Design review of the part built by this model. Coordinates are the model's own, in mm. Coordinates: 2 decimals unless noted, no trailing zeros. Loops run counter-clockwise (first coordinate to the right, second up) from the corner with the lowest first, then second, coordinate; pieces in that order, holes last. Notation, with made-up numbers: (9, 31) - (29, 31) arc R31 ccw to (29, 68) - close; hole circle Ø9 at (89, -39). An arc over 180 degrees is marked (long way). Answer in a Markdown table with one row per item. Add a question column.
(1) We need section A-A, the plane z = 2.5. Give the number of separate pieces and of enclosed holes in the cut face, plus the area to 3 significant figures.
(2) The part is to be moulded in two halves that separate along Y. For faces 1 (the face through (48, -48, 10)), 2 (the face through (50, 39.979, 5)), 3 (the face through (106.06, 9.77, 4.93)), say which applies: released by +Y, released by -Y, zero draft, split by the parting line, or undercut.
(3) To check wall thickness, follow L1, parallel to X at y = -23, z = 9.25; L2, parallel to X at y = -48.5, z = 7.25; L3, parallel to Y at x = -9, z = 0.75. State the ranges of each line that lie inside material, in increasing order. Write a range as [from, to].
(4) Clearance check with flat-ended pins moving along their axes: pin 1 (5 mm diameter, centred on x = -10, y = -6.5, fed in from -Z); pin 2 (5 mm diameter, centred on x = 109.23, y = -109.52, fed in from -Z); pin 3 (11 mm diameter, centred on x = 49.23, y = -69.52, fed in from +Z); pin 4 (10 mm diameter, centred on x = 49.23, y = -29.52, fed in from +Z). State where each tip first meets the part, or that it passes through.
(5) We need section B-B, the plane y = -52.5. Write out the cut boundary in (x, z), plus the area to 3 significant figures.
Solid Edge part; units mm, degrees
sketch "Sketch1" plane through (0, 0, 0) normal (0, 0, 1) x (1, 0, 0)
  line L0 (-25.7684, -139.0211) -> (124.2316, -139.0211)
  line L1 (124.2316, -139.0211) -> (124.2316, 39.9789)
  line L2 (124.2316, 39.9789) -> (-25.7684, 39.9789)
  line L3 (-25.7684, 39.9789) -> (-25.7684, -139.0211)
extrude "Protrusion1" add sketch "Sketch1" along normal blind 10
sketch "Sketch2" plane through (49.2316, -49.5211, 10) normal (0, 0, 1) x (0, -1, 0)
  circle A0 centre (0, 45) radius 15
extrude "Cutout1" cut sketch "Sketch2" against normal through all
hole "Hole_1" at (49.2316, -29.5211, 10) direction (0, 0, -1) diameter 8.5 end up to next countersink diameter 18 countersink angle 90
hole "Hole1" at (109.2316, -29.5211, 10) direction (0, 0, -1) diameter 8.5 end up to next countersink diameter 18 countersink angle 90
hole "Hole2" at (109.2316, -69.5211, 10) direction (0, 0, -1) diameter 8.5 end up to next countersink diameter 18 countersink angle 90
hole "Hole3" at (49.2316, -69.5211, 10) direction (0, 0, -1) diameter 8.5 end up to next countersink diameter 18 countersink angle 90
hole "Hole4" at (-10.7684, -69.5211, 10) direction (0, 0, -1) diameter 8.5 end up to next countersink diameter 18 countersink angle 90
hole "Hole5" at (-10.7684, -29.5211, 10) direction (0, 0, -1) diameter 8.5 end up to next countersink diameter 18 countersink angle 90
hole "Hole_7" at (49.2316, -109.5211, 0) direction (0, 0, 1) diameter 6.5 end up to next
hole "Hole6" at (-10.7684, -109.5211, 0) direction (0, 0, 1) diameter 6.5 end up to next
hole "Hole7" at (-10.7684, 10.4789, 0) direction (0, 0, 1) diameter 6.5 end up to next
hole "Hole8" at (49.2316, 10.4789, 0) direction (0, 0, 1) diameter 6.5 end up to next
hole "Hole9" at (109.2316, 10.4789, 0) direction (0, 0, 1) diameter 6.5 end up to next
hole "Hole10" at (109.2316, -109.5211, 0) direction (0, 0, 1) diameter 6.5 end up to next
properties material "Aluminum, 6061-T6"
Responses:
| question | item | result |
|---|---|---|
| 1 | separate pieces | 1 |
| 1 | enclosed holes | 13 |
| 1 | area | 25,600 mm2 |
| 2 | face 1 | zero draft |
| 2 | face 2 | released by +Y |
| 2 | face 3 | undercut |
| 3 | L1 | x = [-25.77, -15.82], [-5.71, 44.18], [54.29, 104.18], [114.29, 124.23] |
| 3 | L2 | x = [-25.77, 79.27], [109.2, 124.23] |
| 3 | L3 | y = [-139.02, -112.25], [-106.79, -73.39], [-65.66, -33.39], [-25.66, 7.75], [13.21, 39.98] |
| 4 | pin 1 | stops at z = 0 |
| 4 | pin 2 | passes through |
| 4 | pin 3 | stops at z = 6.5 |
| 4 | pin 4 | stops at z = 6 |
| 5 | outline | (-25.77, 0) - (79.53, 0) - (79.53, 10) - (-25.77, 10) - close; (108.93, 0) - (124.23, 0) - (124.23, 10) - (108.93, 10) - close |
| 5 | area | 1,210 mm2 |
